Geometry: see drawing. Coordinates: mm, zero at the bounding-box minimum. A direction names the side the tool comes from. Give positions to 0.01 mm unless a question says otherwise; leave off trailing zeros. Loops run counter-clockwise (first coordinate to the right, second up) from the corner with the lowest first, then second, coordinate; pieces in that order, holes last. Notation, with made-up numbers: (83, -36.75) -> (122, -36.75) arc R28 cw to (122, -1.75) -> close; hole circle Ø4 at (78, 32.25). An arc over 180 degrees is marked (long way). Return JSON: item names as keys, results as strings. Group by question number.
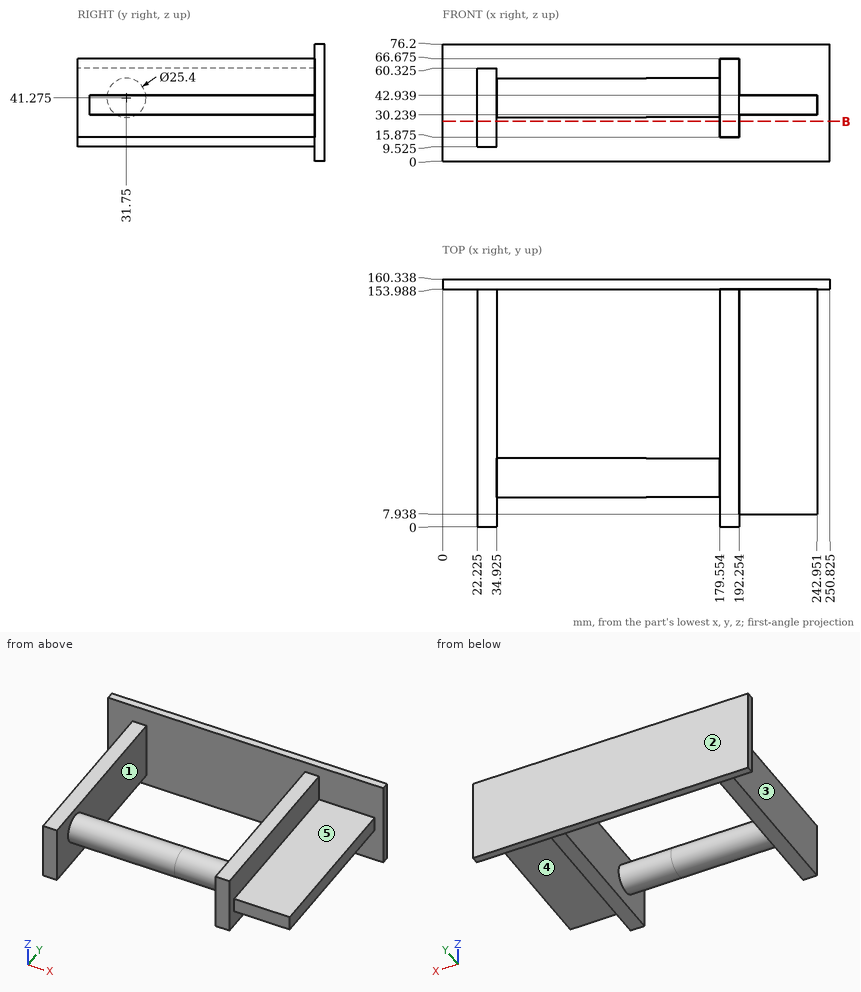
1) Cut plane B-B on z = 26. Return loops of the section in (x, y) (1 decimal).
2) Mould query, pull axis X, two halves, no side actions, for the marked faces 1, 2 and 3. Classes: released by +X, released by -X, zero draft, split by the parting line, or undercut.
3) Contact query for flat-ended pins moving along their axis: P1, Ø10, axis at x = 27, y = 84, coming from the -Z side (1 decimal); P2, Ø3, axis at x = 88, z = 48.5, coming from the -Y side; P3, Ø6, axis at x = 211, y = 18.5, coming from the -Z side. Output: stop coordinate, or through.
4) Reachability of the marked faces 4 and 5 from +Z, -Z, +X, -X, +Y, -Y: full face, straight path, thin tool, end or side. Return the list, or none.
5) Material intervals for line 1 (X direction, y = 59, z = 21) (1 decimal); line 2 (Z direction, x = 194, y = 153); line 3 (Y direction, x = 89.5, z = 28.5), sorted ascending.
Calculated:
{
 "1": {"outline": "(0, 154) -> (22.2, 154) -> (22.2, 0) -> (34.9, 0) -> (34.9, 154) -> (179.6, 154) -> (179.6, 0) -> (192.3, 0) -> (192.3, 154) -> (250.8, 154) -> (250.8, 160.3) -> (0, 160.3) -> close"},
 "2": {"face 1": "undercut", "face 2": "zero draft", "face 3": "released by -X"},
 "3": {"P1": "z = 9.5", "P2": "y = 20.41", "P3": "z = 30.24"},
 "4": {"face 4": "-Z, +X, -Y", "face 5": "+Z, +X, -Y"},
 "5": {"line 1": "22.2 to 34.9, 179.6 to 192.3", "line 2": "30.24 to 42.94", "line 3": "153.99 to 160.34"}
}
